Verification items for the finished model (mm, model axes). Face numbers are marked on the shaded views. Round coordinates to 2 decimals unless told otherwise and drop trailing zeros. Write each loop counter-clockwise with the first axis right and the second up, starting at its lowest first coordinate (ties: lowest second). Pieces come first, ordered by that corner, then holes.
Autodesk Inventor part; units mm, degrees
ref_plane "YZ Plane" through (0, 0, 0) normal (1, 0, 0) x (0, 1, 0)
ref_plane "XZ Plane" through (0, 0, 0) normal (0, 1, 0) x (-1, 0, 0)
ref_plane "XY Plane" through (0, 0, 0) normal (0, 0, 1) x (1, 0, 0)
sketch "Sketch1" plane through (0, 0, 0) normal (0, 1, 0) x (-1, 0, 0)
  line L0 (0, 0) -> (35, 0)
  line L1 (35, 0) -> (35, 6)
  line L2 (0, 6) -> (35, 6)
  line L3 (0, 0) -> (0, 6)
  line L4 (0, 6) -> (0, 0)
  line L5 (0, 3) -> (35, 3)
  line L6 (17.5, 3) -> (35, 3)
  line L7 (17.5, 3) -> (0, 3)
  point P0 (17.5, 0)
  point P1 (8.75, 3)
  point P2 (26.25, 3)
extrude "Extrusion1" add sketch "Sketch1" along normal blind 5
sketch "Sketch2" plane through (-35, 0, 6) normal (0, 0, 1) x (1, 0, 0)
  line L0 (0, 0) -> (35, 0)
  line L1 (35, 0) -> (35, 5)
  line L2 (0, 5) -> (35, 5)
  line L3 (0, 0) -> (0, 5)
extrude "Extrusion2" add sketch "Sketch2" along normal blind 30
sketch "Sketch3" plane through (0, 5, 0) normal (0, 1, 0) x (1, 0, 0)
  line L0 (0, 0) -> (0, -36)
  line L1 (0, 0) -> (-35, 0)
  line L2 (-35, 0) -> (-35, -36)
  line L3 (0, -36) -> (-35, -36)
  line L4 (-35, 0) -> (-35, -36)
  line L5 (-35, -31) -> (0, -31)
  line L6 (0, -31) -> (0, -25)
  line L7 (0, -25) -> (-35, -25)
  line L8 (-35, -25) -> (-35, -31)
  dimension "d4" = 5
  dimension "d5" = 25
sketch "Sketch4" plane through (0, 0, 0) normal (0, -1, 0) x (1, 0, 0)
  line L0 (-35, 0) -> (0, 0)
  line L1 (0, 0) -> (0, 6)
  line L2 (-35, 6) -> (0, 6)
  line L3 (-35, 0) -> (-35, 6)
  line L4 (-35, 6) -> (-35, 0)
  line L5 (-35, 3) -> (0, 3)
  line L6 (-17.5, 3) -> (0, 3)
  line L7 (-17.5, 3) -> (-35, 3)
  point P0 (0, 0)
  point P1 (-17.5, 0)
  point P2 (-8.75, 3)
  point P3 (-26.25, 3)
hole "Hole1" at (-8.75, 0, 3) at (-26.25, 0, 3) direction (0, 1, 0) diameter 3 depth 8 tip angle 118
sketch "Sketch5" plane through (0, 5, 0) normal (0, 1, 0) x (1, 0, 0)
  line L0 (-99.5, -29.2319) -> (64.2547, -8.9987)
  line L1 (64.5, -10.9836) -> (-99.2547, -31.2168)
  line L2 (0, -20.4645) -> (-35, -24.789)
  line L3 (-35, -19.751) -> (0, -15.4265)
  line L4 (0, -15.4265) -> (0, -20.4645)
  line L5 (-35, -19.751) -> (-35, -24.789)
  dimension "d15" = 1.5
  dimension "d16" = 1.5
extrude "Extrusion4" cut sketch "Sketch5" against normal blind 2
sketch "Sketch7" plane through (0, 5, 0) normal (0, 1, 0) x (1, 0, 0)
  line L0 (0, -15.4265) -> (0, -20.4645)
  line L1 (0, -19.751) -> (0, -24.789)
  line L2 (-35, 0) -> (-35, -36)
  line L3 (-35, -36) -> (-35, -49.8548)
  line L4 (-35, -20.4645) -> (0, -24.789)
  line L5 (0, -19.751) -> (-35, -15.4265)
  line L6 (-35, -15.4265) -> (-35, -20.4645)
  line L7 (0, 0) -> (0, -36)
extrude "Extrusion5" cut sketch "Sketch7" against normal blind 2
properties part number "side_clip" material "ABS Plastic"
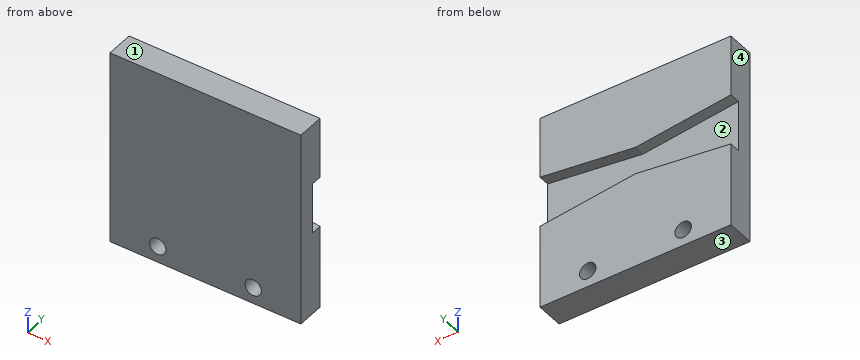
Q1. Release check for a two-part mould opening along Z. For the marked faces 1, 2, 3 and 4 record: released by +Z, released by -Z, zero draft, split by the parting line, or undercut.
Recorded:
face 1: released by +Z
face 2: undercut
face 3: released by -Z
face 4: zero draft
Q2. Sectioned sample at C-C (z = 19). Enter the section's corners in (x, y), plus the area to 3 significant figures.
Recorded:
outline: (-35, 0) - (0, 0) - (0, 3) - (-35, 3) - close
area: 105 mm2
Q3. Depth check by flat-ended pin: P1, Ø1.5, axis at x = -13, z = 11.5, coming from the -Y side; P2, Ø4.5, axis at x = -24, z = 21, coming from the +Y side. Enter the tip coordinate at first touch or a pass-through.
Recorded:
P1: stops at y = 0
P2: stops at y = 3
Q4. Sectioned sample at B-B (x = -26.25). Enter the section's corners in (y, z).
Recorded:
outline: (0, 0) - (5, 0) - (5, 1.5) - (0, 1.5) - close; (0, 4.5) - (5, 4.5) - (5, 16.51) - (3, 16.51) - (3, 23.71) - (5, 23.71) - (5, 36) - (0, 36) - close
Q5. Material ranges on line 1 along X through (y, z) = (2.6, 3); line 2 along Z through (x, y) = (-26.25, 2.8); line 3 along Z through (x, y) = (-25, 3.45), recorded low to high.
Recorded:
line 1: x = -35 to -27.75, -24.75 to -10.25, -7.25 to 0
line 2: z = 0 to 1.5, 4.5 to 36
line 3: z = 0 to 2.17, 3.83 to 16.66, 23.55 to 36
Q6. Sectioned sample at A-A (z = 3). Enter the section's corners in (x, y), plus the area to 3 significant figures.
Recorded:
outline: (-35, 0) - (-27.75, 0) - (-27.75, 5) - (-35, 5) - close; (-24.75, 0) - (-10.25, 0) - (-10.25, 5) - (-24.75, 5) - close; (-7.25, 0) - (0, 0) - (0, 5) - (-7.25, 5) - close
area: 145 mm2
